CAD build for the part. Positions are in the model's coordinates, mm. A direction names the side the tool comes from. Give positions to 0.01 mm unless a question says otherwise; leave off trailing zeros. Write each loop counter-clockwise with the first axis right and the second up, starting at its lowest first coordinate (ties: lowest second). Pieces come first, ordered by that corner, then holes. Notation, with made-up numbers: (-2, 0.25) - (26, 0.25) arc R21 cw to (26, 8.25) - close; hole circle Ø1 at (-11, -14). An arc over 180 degrees is marked (long way). Put each result on its own line as item: value. Start each with the question number.
1. Wall check: line 1 (Y direction, x = 24, z = 14); line 2 (Y direction, x = -31, z = 0); line 3 (X direction, y = 10.25, z = -15.5). Give the ranges that are in metal, low to high.
2. Tool access for faces 1 (the flat face through (-42.5, 6, 0)), 2 (the flat face through (17, 10.5, 0)), 3 (the flat face through (-31, 12, 0)): list every direction of +Z, -Z, +X, -X, +Y, -Y with a clear straight run to the whole face (end or side of a thin tool).
3. Mould opens along Z. For faces 4 (the flat face through (-1, 5, -22)), 5 (the flat face through (-32.416, 12.254, 1.267)), 6 (the flat face through (-1, 5, 22)), 7 (the flat face through (-1, 0, 0)) say: +Z half, -Z half, draft (parallel to the pull), parting line (faces both ways), or undercut.
4. Drop a flat-ended pin along its axis: pin 1 (6 mm diameter, centred on x = 27, z = 16, fed in from +Y). Give the stop position or say it passes through.
5. Cut at A-A on x = 34.5. List the corners of the cut face in (y, z).
from build123d import *

# Parameters (mm, degrees)
SKETCH1_W               = 85
SKETCH1_H               = 44
BOSS_EXTRUDE1_DEPTH     = 15
CUT_EXTRUDE1_DEPTH      = 51.152268144
CUT_EXTRUDE1_DEPTH_BACK = 51.152268144
FILLET1_R               = 1
FILLET2_R               = 0.5
FILLET3_R               = 0.5
CUT_EXTRUDE3_DEPTH      = 0.5


with BuildPart() as part:
    # Sketch1 → Boss-Extrude1 (new body)
    with BuildSketch(Plane(origin=(0, 0, 0), x_dir=(1, 0, 0), z_dir=(0, 1, 0))):
        Rectangle(SKETCH1_W, SKETCH1_H)
    extrude(amount=BOSS_EXTRUDE1_DEPTH)

    # Sketch2 → Cut-Extrude1 (cut, two sides: drawn at the far end of the back side and taken through both)
    with BuildSketch(Plane.XY.offset(-CUT_EXTRUDE1_DEPTH_BACK)):
        with BuildLine():
            Line((-42.5, 12.5), (-12.5, 12.5))
            add(Edge.make_bspline(
                [(-12.5, 12.5), (-10.623415355, 12.323006837), (-9.376584645, 10.676993163), (-7.5, 10.5)],
                knots=[0, 0, 0, 0, 1, 1, 1, 1], degree=3))
            Line((-7.5, 10.5), (42.5, 10.5))
            Line((42.5, 10.5), (42.5, 22.5))
            Line((42.5, 22.5), (-42.5, 22.5))
            Line((-42.5, 22.5), (-42.5, 12.5))
        make_face()
    extrude(amount=CUT_EXTRUDE1_DEPTH + CUT_EXTRUDE1_DEPTH_BACK, mode=Mode.SUBTRACT)

    # Fillet1
    fillet1_edges = [part.edges().sort_by_distance(p)[0] for p in [
        (42.5, 5.25, -22),
        (42.5, 5.25, 22),
        (-42.5, 6.25, 22),
        (-42.5, 6.25, -22),
    ]]
    fillet(fillet1_edges, radius=FILLET1_R)

    # Fillet2
    fillet2_edges = [part.edges().sort_by_distance(p)[0] for p in [
        (17, 10.5, -22),
        (-9.999999993, 11.50000001, -22),
        (-9.999999993, 11.50000001, 22),
        (17, 10.5, 22),
        (-42.5, 12.5, 0),
        (-27, 12.5, -22),
        (-27, 12.5, 22),
        (-42.207106781, 12.5, 21.707106781),
        (-42.207106781, 12.5, -21.707106781),
        (42.5, 10.5, 0),
        (42.207106781, 10.5, 21.707106781),
        (42.207106781, 10.5, -21.707106781),
    ]]
    fillet(fillet2_edges, radius=FILLET2_R)

    # Fillet3
    fillet3_edges = [part.edges().sort_by_distance(p)[0] for p in [
        (-42.5, 0, 0),
        (0, 0, -22),
        (42.5, 0, 0),
        (0, 0, 22),
        (-42.207106781, 0, 21.707106781),
        (42.207106781, 0, 21.707106781),
        (42.207106781, 0, -21.707106781),
        (-42.207106781, 0, -21.707106781),
    ]]
    fillet(fillet3_edges, radius=FILLET3_R)

    # Sketch4 → Cut-Extrude3 (cut)
    with BuildSketch(Plane(origin=(0, 12.5, 0), x_dir=(1, 0, 0), z_dir=(0, 1, 0))):
        Polygon((-38.5, 0), (-26.5, 2.5), (-26.5, -2.5), align=None)
    extrude(amount=-CUT_EXTRUDE3_DEPTH, mode=Mode.SUBTRACT)


solid = part.part
Report:
1. line 1: y = 0 to 10.5
1. line 2: y = 0 to 12
1. line 3: x = -42.5 to 42.43
2. face 1: +Z, -Z, -X, +Y, -Y
2. face 2: +Z, -Z, +X, +Y
2. face 3: +Y
3. face 4: -Z half
3. face 5: undercut
3. face 6: +Z half
3. face 7: draft
4. pin 1: stops at y = 10.5
5. outline: (0, -21.5) arc R0.5 ccw to (0.5, -22) - (10, -22) arc R0.5 ccw to (10.5, -21.5) - (10.5, 21.5) arc R0.5 ccw to (10, 22) - (0.5, 22) arc R0.5 ccw to (0, 21.5) - close
